```python
from build123d import *

# Parameters (mm, degrees)
BOSS_EXTRUDE1_DEPTH  = 52.09999994
BOSS_EXTRUDE2_START  = -52.09999994
SKETCH2_R            = 3
BOSS_EXTRUDE2_DEPTH  = 52.09999994
FILLET1_R            = 2.54
FILLET2_R            = 1.27
FILLET2_OF_MIRROR1_R = 1.27
FILLET3_R            = 1.27
FILLET4_R            = 2.54


with BuildPart() as part:
    # Sketch1 → Boss-Extrude1 (new body)
    with BuildSketch(Plane(origin=(0, 0, 0), x_dir=(1, 0, 0), z_dir=(0, 1, 0))):
        with BuildLine():
            Line((0, 120.3706), (0, 0))
            Line((0, 0), (3.175, 0))
            Line((3.175, 0), (3.175, 120.3706))
            ThreePointArc((3.175, 120.3706), (5.220859133, 125.309740867), (10.16, 127.3556))
            Line((10.16, 127.3556), (20.32, 127.3556))
            Line((20.32, 127.3556), (20.32, 130.5306))
            Line((20.32, 130.5306), (10.16, 130.5306))
            ThreePointArc((10.16, 130.5306), (2.975795103, 127.554804897), (0, 120.3706))
        make_face()
        with BuildLine():
            Line((3.175, 0), (0, 0))
            ThreePointArc((0, 0), (2.975795103, -7.184204897), (10.16, -10.16))
            Line((10.16, -10.16), (20.32, -10.16))
            Line((20.32, -10.16), (20.32, -6.985))
            Line((20.32, -6.985), (10.16, -6.985))
            ThreePointArc((10.16, -6.985), (5.220859133, -4.939140867), (3.175, 0))
        make_face()
    extrude(amount=BOSS_EXTRUDE1_DEPTH)

    # Sketch2 → Boss-Extrude2 (add)
    with BuildSketch(Plane(origin=(0, 52.09999994, 0), x_dir=(1, 0, 0), z_dir=(0, 1, 0)).offset(BOSS_EXTRUDE2_START)):
        with BuildLine():
            Line((3.175, 112.856959641), (10.16, 112.856959641))
            Line((10.16, 112.856959641), (20.32, 112.856959641))
            Line((20.32, 112.856959641), (20.32, 127.3556))
            Line((20.32, 127.3556), (10.16, 127.3556))
            ThreePointArc((10.16, 127.3556), (5.220859133, 125.309740867), (3.175, 120.3706))
            Line((3.175, 120.3706), (3.175, 112.856959641))
        make_face()
        with Locations(Location((14.1478, 120.3706, 0), (0, 0, 270))):
            Circle(SKETCH2_R, mode=Mode.SUBTRACT)
    boss_extrude2 = extrude(amount=BOSS_EXTRUDE2_DEPTH)

    # Fillet1
    fillet1_edges = [part.edges().sort_by_distance(p)[0] for p in [
        (20.32, 26.04999997, -112.856959641),
    ]]
    fillet(fillet1_edges, radius=FILLET1_R)

    # Fillet2
    fillet2_edges = [part.edges().sort_by_distance(p)[0] for p in [
        (3.175, 26.04999997, -112.856959641),
    ]]
    fillet(fillet2_edges, radius=FILLET2_R)

    # Mirror1: Boss-Extrude2 across plane
    add(boss_extrude2.mirror(Plane(origin=(0, 0, -60.1853), x_dir=(1, 0, 0), z_dir=(0, 0, -1))))

    # Fillet2 of Mirror1
    fillet2_of_mirror1_edges = [part.edges().sort_by_distance(p)[0] for p in [
        (3.175, 26.04999997, -7.513640359),
    ]]
    fillet(fillet2_of_mirror1_edges, radius=FILLET2_OF_MIRROR1_R)

    # Fillet3
    fillet3_edges = [part.edges().sort_by_distance(p)[0] for p in [
        (20.32, 26.04999997, 10.16),
        (20.32, 26.04999997, -130.5306),
    ]]
    fillet(fillet3_edges, radius=FILLET3_R)

    # Fillet4
    fillet4_edges = [part.edges().sort_by_distance(p)[0] for p in [
        (20.32, 26.04999997, -7.513640359),
    ]]
    fillet(fillet4_edges, radius=FILLET4_R)


solid = part.part
```
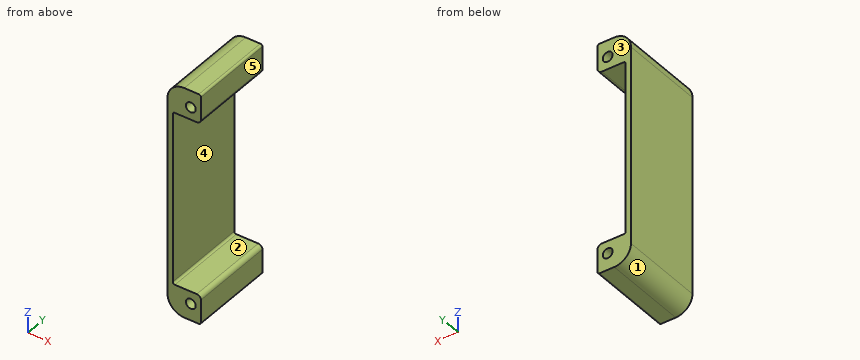
For this review, take the finished solid that the model builds, in its own axes (mm). Face numbers are marked on the shaded views. A direction names the side the tool comes from. Give positions to 0.01 mm unless a question says otherwise; leave off trailing zeros. Order: outer loops, then holes, each group sorted by start corner. A loop starts at its lowest first (then second) coordinate and runs counter-clockwise, first axis right, second up.
1) Take a section at A-A (x = 12.5). Give the boundary of the cut face in (y, z).
2) Take a section at C-C (z = -53). Give the boundary of the cut face in (x, y) (3 decimals).
3) Insertion check: pin 1 (1.5 mm diameter, centred on y = 34.5, z = -71, fed in from +X) (3 decimals); pin 2 (3 mm diameter, centred on x = 4, y = 14.5, fed in from +Z); pin 3 (5.5 mm diameter, centred on x = 14.15, z = -120.37, fed in from +Y). Each pin has a flat end and moves straight along its axis. Give the tip position at first contact, or say it passes through.
4) Take a section at B-B (y = 8). Give the boundary of the cut face in (x, z) (3 decimals), then the cut area to 3 significant figures.
5) Wall thickness on line 1 (Z direction, x = 14.5, y = 23); line 2 (Z direction, x = 14.25, y = 8); line 3 (Z direction, x = 17.75, y = 14): over which ranges is each line inside the solid? List them lowest first.
6) For the marked faces 4 and 5, list the 3-axis set-ups (+Z, -Z, +X, -X, +Y, -Y) from which the entire face can be reached by the end or side of a thin tool; tool diameter is ignored.
7) The part is to be moulded in two halves that separate along Z. For the marked faces 1, 2 and 3, say which applies: released by +Z, released by -Z, zero draft, split by the parting line, or undercut.
Derived:
1. outline: (0, -130.53) - (52.1, -130.53) - (52.1, -122.88) - (0, -122.88) - close; (0, -117.86) - (52.1, -117.86) - (52.1, -112.86) - (0, -112.86) - close; (0, -7.51) - (52.1, -7.51) - (52.1, -2.51) - (0, -2.51) - close; (0, 2.51) - (52.1, 2.51) - (52.1, 10.16) - (0, 10.16) - close
2. outline: (0, 0) - (3.175, 0) - (3.175, 52.1) - (0, 52.1) - close
3. pin 1: stops at x = 3.175
3. pin 2: stops at z = 9.03
3. pin 3: passes through
4. outline: (0, -120.371) arc R10.16 ccw to (10.16, -130.531) - (19.05, -130.531) arc R1.27 ccw to (20.32, -129.261) - (20.32, -115.397) arc R2.54 ccw to (17.78, -112.857) - (4.445, -112.857) arc R1.27 cw to (3.175, -111.587) - (3.175, -8.784) arc R1.27 cw to (4.445, -7.514) - (17.78, -7.514) arc R2.54 ccw to (20.32, -4.974) - (20.32, 8.89) arc R1.27 ccw to (19.05, 10.16) - (10.16, 10.16) arc R10.16 ccw to (0, 0) - close; hole circle Ø6 at (14.148, -120.371); hole circle Ø6 at (14.148, 0)
4. area: 949 mm2
5. line 1: z = -130.53 to -123.35, -117.39 to -112.86, -7.51 to -2.98, 2.98 to 10.16
5. line 2: z = -130.53 to -123.37, -117.37 to -112.86, -7.51 to -3, 3 to 10.16
5. line 3: z = -130.53 to -112.86, -7.51 to 10.16
6. face 4: +X, +Y, -Y
6. face 5: +Z, -Z, +X, +Y, -Y
7. face 1: released by -Z
7. face 2: undercut
7. face 3: zero draft
